```python
from build123d import *

# Parameters (mm, degrees)
SKETCH1_R               = 10
BOSS_EXTRUDE1_DEPTH     = 120
SKETCH4_R               = 6
CUT_EXTRUDE3_DEPTH      = 40
CUT_EXTRUDE3_DEPTH_BACK = 40
SKETCH5_W               = 23.593926408
SKETCH5_H               = 33.705609154
CUT_EXTRUDE4_DEPTH      = 4
CUT_EXTRUDE4_DEPTH_BACK = 4


with BuildPart() as part:
    # Sketch1 → Boss-Extrude1 (new body)
    with BuildSketch(Plane(origin=(0, 0, 0), x_dir=(0, 1, 0), z_dir=(0, 0, 1))):
        Circle(SKETCH1_R)
    extrude(amount=BOSS_EXTRUDE1_DEPTH)

    # Sketch4 → Cut-Extrude3 (cut, two sides)
    with BuildSketch(Plane.YZ) as cut_extrude3_sk:
        with Locations((0, 14)):
            Circle(SKETCH4_R)
    extrude(amount=CUT_EXTRUDE3_DEPTH, mode=Mode.SUBTRACT)
    extrude(cut_extrude3_sk.sketch, amount=-CUT_EXTRUDE3_DEPTH_BACK, mode=Mode.SUBTRACT)

    # Sketch5 → Cut-Extrude4 (cut, two sides)
    with BuildSketch(Plane.YZ) as cut_extrude4_sk:
        with Locations((0.674112183, 13.2334673)):
            Rectangle(SKETCH5_W, SKETCH5_H)
    extrude(amount=CUT_EXTRUDE4_DEPTH, mode=Mode.SUBTRACT)
    extrude(cut_extrude4_sk.sketch, amount=-CUT_EXTRUDE4_DEPTH_BACK, mode=Mode.SUBTRACT)


solid = part.part
```
Part model, mm, in its own coordinate system. A direction names the side the tool comes from. Give positions to 0.01 mm unless a question says otherwise; leave off trailing zeros. Order: outer loops, then holes, each group sorted by start corner. A loop starts at its lowest first (then second) coordinate and runs counter-clockwise, first axis right, second up. Notation, with made-up numbers: (51, 5.25) - (106, 5.25) arc R21 cw to (106, 26.25) - close; hole circle Ø6 at (87.5, 24). An arc over 180 degrees is marked (long way). Use one line per item in the form item = value.
Item 1: Probe probe 1 along Z at (x, y) = (5.75, 0); probe 2 along Z at (x, y) = (3.75, 4.5); probe 3 along X at (y, z) = (-3.5, 21.5). List the from-to ranges inside material, lowest first. Write a range as from..to.
Solution:
probe_1 = 0..8, 20..120
probe_2 = 30.09..120
probe_3 = -9.37..-4, 4..9.37
Item 2: Slice it at C-C on y = 7.5. Give the cut face in (x, z), and give its area (3 significant figures).
Solution:
outline = (-6.61, 0) - (-4, 0) - (-4, 30.09) - (4, 30.09) - (4, 0) - (6.61, 0) - (6.61, 120) - (-6.61, 120) - close
area = 1,350 mm2
Item 3: Slice it at D-D on z = 89. Give the cut face in (x, y), and give its area (3 significant figures).
Solution:
outline = circle Ø20 at (0, 0)
area = 314 mm2
Item 4: Slice it at A-A on z = 14. Give the cut face in (x, y), and give its area (3 significant figures).
Solution:
outline = (-8, -6) arc R10 ccw to (-4, -9.17) - (-4, -6) - close; (-8, 6) - (-4, 6) - (-4, 9.17) arc R10 ccw to start; (4, -9.17) arc R10 ccw to (8, -6) - (4, -6) - close; (4, 6) - (8, 6) arc R10 ccw to (4, 9.17) - close
area = 29.8 mm2
Item 5: Two-plate mould, pull along X, no slides. Class faces 3 (the face through (0, 0, 30.086)), 4 (the face through (0, -10, 59)), 5 (the face through (6, 0, 0)): released by +X, released by -X, zero draft, split by the parting line, or undercut.
Solution:
face_3 = undercut
face_4 = split by the parting line
face_5 = zero draft
Item 6: Which spindle directions (+Z, -Z, +X, -X, +Y, -Y) get a long thin tool onto all of the face, cutting with end or side? Do faces 1 (the face through (-4, 4, 19)), 2 (the face through (6.297, 2.769, 8.677)). Say none if no direction does.
Solution:
face_1 = -Z, +Y, -Y
face_2 = +X, -X
Item 7: Pin check, flat tips, straight feed: pin 1 Ø4 at (y, z) = (5, 16.5) entering from -X; pin 2 Ø8 at (y, z) = (-5.5, 84.5) entering from -X; pin 3 Ø2 at (x, z) = (2, 104) entering from +Y; pin 4 Ø11 at (y, z) = (0, 14) entering from +X. Stop position of each tip, or through.
Solution:
pin_1 = -9.09
pin_2 = -9.89
pin_3 = 9.95
pin_4 = through
Item 8: Slice it at B-B on y = -2.75. Give the cut face in (x, z), and give its area (3 significant figures).
Solution:
outline = (-9.61, 0) - (-4, 0) - (-4, 8.67) - (-9.61, 8.67) - close; (-9.61, 19.33) - (-4, 19.33) - (-4, 30.09) - (4, 30.09) - (4, 19.33) - (9.61, 19.33) - (9.61, 120) - (-9.61, 120) - close; (4, 0) - (9.61, 0) - (9.61, 8.67) - (4, 8.67) - close
area = 1,950 mm2
